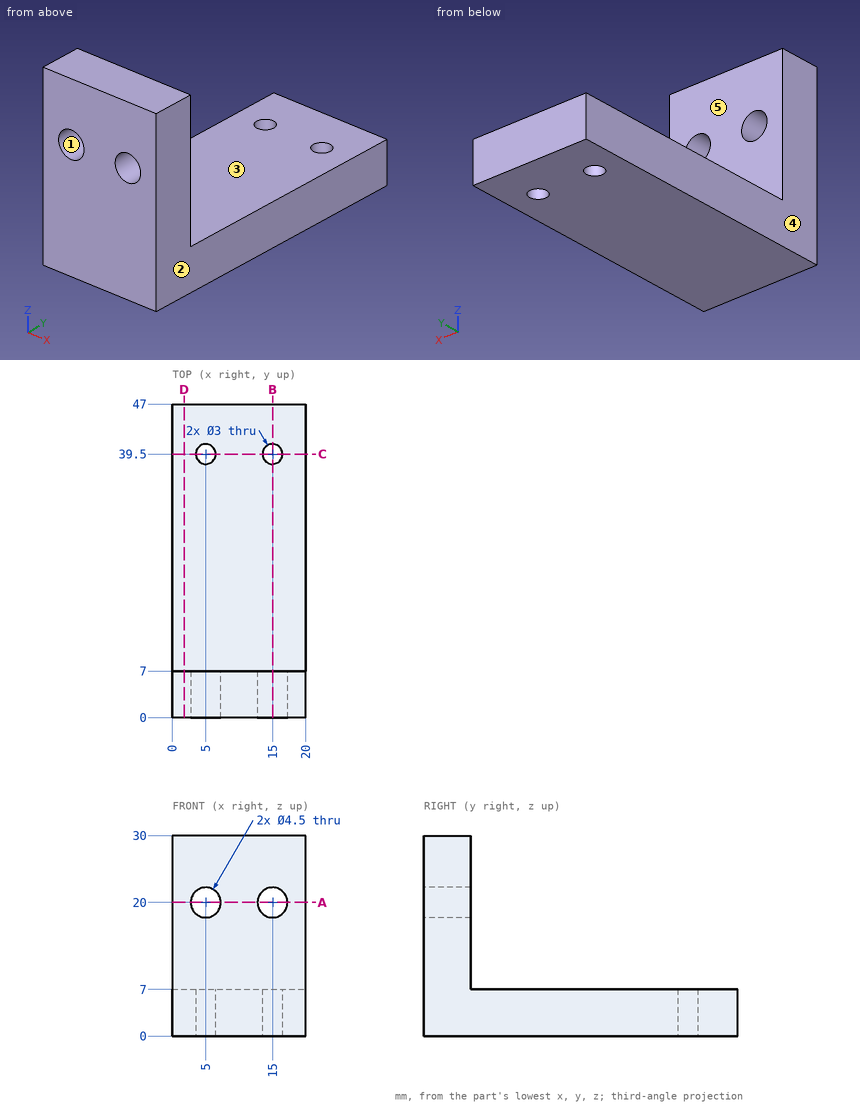
Print and shaded views of the part. All mm, measured from the part's lowest x, y and z. A direction names the side the tool comes from. Round coordinates to 2 decimals unless told otherwise and drop trailing zeros. Write each loop counter-clockwise with the first axis right and the second up, starting at its lowest first coordinate (ties: lowest second). Pieces come first, ordered by that corner, then holes. Notation, with made-up numbers: (9, 19.25) - (23, 19.25) arc R16 cw to (23, 31.25) - close; hole circle Ø5 at (39.5, 29). An arc over 180 degrees is marked (long way). Write each question's results on one line, items separated by ' | '. Start each with the question number.
Item 1: Wall check: L1, parallel to Z at x = 5, y = 2.75; L2, parallel to Y at x = 15, z = 3; L3, parallel to Z at x = 18, y = 26. Give the ranges that are in metal, low to high. Write a range as [from, to].
Item 2: Which spindle directions (+Z, -Z, +X, -X, +Y, -Y) get a long thin tool onto all of the face, cutting with end or side? Do the marked faces 4 and 5. Say none if no direction does.
Item 3: Saw through at C-C (y = 39.5). Write the cut outline in (x, z), and give its area (3 significant figures).
Item 4: Drop flat-ended pins along their axis: P1, Ø4, axis at x = 7, y = 21, coming from the +Z side; P2, Ø7, axis at x = 15, z = 20, coming from the +Y side; P3, Ø1.8, axis at x = 15, y = 39.5, coming from the +Z side. Give the stop position or say it passes through.
Item 5: Saw through at D-D (x = 1.75). Write the cut outline in (y, z).
Item 6: Mould opens along X. For the marked faces 1, 2 and 3 say: pulls with the +X half, pulls with the -X half, needs draft (parallel to the pull), parting line crosses it, or undercut.
Item 7: Saw through at B-B (x = 15). Write the cut outline in (y, z).
Item 8: Saw through at A-A (z = 20). Write the cut outline in (x, y).
Results are:
1) L1: z = [0, 17.75], [22.25, 30] | L2: y = [0, 38], [41, 47] | L3: z = [0, 7]
2) face 4: +Z, -Z, -X, +Y, -Y | face 5: +Z, +X, -X, +Y
3) outline: (0, 0) - (3.5, 0) - (3.5, 7) - (0, 7) - close; (6.5, 0) - (13.5, 0) - (13.5, 7) - (6.5, 7) - close; (16.5, 0) - (20, 0) - (20, 7) - (16.5, 7) - close | area: 98.0 mm²
4) P1: stops at z = 7 | P2: stops at y = 7 | P3: passes through
5) outline: (0, 0) - (47, 0) - (47, 7) - (7, 7) - (7, 30) - (0, 30) - close
6) face 1: undercut | face 2: pulls with the +X half | face 3: needs draft
7) outline: (0, 0) - (38, 0) - (38, 7) - (7, 7) - (7, 17.75) - (0, 17.75) - close; (0, 22.25) - (7, 22.25) - (7, 30) - (0, 30) - close; (41, 0) - (47, 0) - (47, 7) - (41, 7) - close
8) outline: (0, 0) - (2.75, 0) - (2.75, 7) - (0, 7) - close; (7.25, 0) - (12.75, 0) - (12.75, 7) - (7.25, 7) - close; (17.25, 0) - (20, 0) - (20, 7) - (17.25, 7) - close
